Autodesk Inventor part; units mm, degrees
ref_plane "YZ Plane" through (0, 0, 0) normal (1, 0, 0) x (0, 1, 0)
ref_plane "XZ Plane" through (0, 0, 0) normal (0, 1, 0) x (-1, 0, 0)
ref_plane "XY Plane" through (0, 0, 0) normal (0, 0, 1) x (1, 0, 0)
sketch "Sketch1" plane through (0, 0, 0) normal (0, 0, 1) x (1, 0, 0)
  line L0 (0, 0) -> (189.177, 0)
  line L1 (189.177, 0) -> (189.177, 325.825)
  line L2 (189.177, 325.825) -> (0, 325.825)
  line L3 (0, 325.825) -> (0, 0)
  dimension "d0" = 189.177
  dimension "d1" = 325.825
extrude "Extrusion1" add sketch "Sketch1" along normal blind 2.6
sketch "Sketch2" plane through (0, 0, 2.6) normal (0, 0, 1) x (1, 0, 0)
  line L0 (0, 325.825) -> (0, 0)
  line L1 (0, 170) -> (0, 0)
  line L2 (0, 170) -> (0, 159.84) construction
  line L3 (0, 159.84) -> (6.35, 159.84) construction
  line L4 (6.35, 170) -> (163.83, 170) construction
  line L5 (163.83, 170) -> (163.83, 136.98) construction
  line L6 (6.35, 159.84) -> (6.35, 4.9) construction
  line L7 (6.35, 4.9) -> (163.83, 4.9) construction
  line L8 (6.35, 159.84) -> (15.9385, 159.84) construction
  line L9 (15.9385, 159.84) -> (15.9385, 4.9) construction
  line L10 (163.83, 136.98) -> (173.4185, 136.98) construction
  line L11 (173.4185, 136.98) -> (173.4185, 4.9) construction
  line L12 (0, 325.825) -> (0, 315.665) construction
  line L13 (15.9385, 159.84) -> (15.9385, 315.665) construction
  line L14 (173.4185, 136.98) -> (173.4185, 292.805) construction
  line L15 (15.9385, 4.9) -> (15.9385, 160.725) construction
  line L16 (173.4185, 4.9) -> (173.4185, 160.725) construction
  circle A0 centre (173.4185, 160.725) radius 1.98
  circle A1 centre (15.9385, 160.725) radius 1.98
  circle A2 centre (15.9385, 315.665) radius 1.98
  circle A3 centre (173.4185, 292.805) radius 1.98
  dimension "d4" = 10.16
  dimension "d6" = 157.48
  dimension "d7" = 33.02
  dimension "d8" = 154.94
  dimension "d13" = 9.5885
  dimension "d14" = 9.5885
  dimension "d19" = 10.16
  dimension "d20" = 155.825
  dimension "d21" = 155.825
  dimension "d22" = 155.825
  dimension "d23" = 3.96
  dimension "d24" = 3.96
  dimension "d25" = 3.96
  dimension "d26" = 3.96
extrude "Extrusion2" cut sketch "Sketch2" against normal blind 5
sketch "Sketch4" plane through (0, 0, 2.6) normal (0, 0, 1) x (1, 0, 0)
  line L0 (0, 0) -> (189.177, 0)
  line L1 (189.177, 0) -> (164.5885, 0) construction
  line L2 (164.5885, 0) -> (24.5885, 0)
  line L3 (24.5885, 0) -> (24.5885, 40)
  line L4 (24.5885, 40) -> (164.5885, 40)
  line L5 (164.5885, 40) -> (164.5885, 0)
  dimension "d29" = 24.5885
  dimension "d30" = 140
  dimension "d31" = 40
extrude "Extrusion3" cut sketch "Sketch4" against normal blind 10
properties part number "trunk"
Geometry check sheet. Reference: the model listing, model coordinates, mm. Coordinates: 2 decimals unless noted, no trailing zeros. Write each loop counter-clockwise with the first axis right and the second up, starting at its lowest first coordinate (ties: lowest second). Pieces come first, ordered by that corner, then holes. Notation, with made-up numbers: M 47.25,76 L 57.25,76 A36 ccw 57.25,115 Z; hole C 51.5,82 d10. An arc over 180 degrees is marked long. One line per item, written item: value. Start each with the question number.
(1) Sectioned sample at B-B, the plane x = 60. Enter the section's corners in (y, z) (3 decimals).
(2) Sectioned sample at A-A, the plane z = 1.7. Enter the section's corners in (x, y) (1 decimal), and give its area (3 significant figures).
(3) Depth check by flat-ended pin: pin 1 (1.3 mm diameter, centred on x = 105, z = 1.5, fed in from -Y). Enter the tip coordinate at first touch or a pass-through.
(4) Scan lines: line 1 along X through (y, z) = (22.5, 2.2); line 2 along Y through (x, z) = (175, 0.6) (3 decimals); line 3 along Y through (x, z) = (33, 0.45) (3 decimals). Record each from-to range of solid material in increasing order. Write a range as [from, to].
Filled sheet:
1. outline: M 40,0 L 325.825,0 L 325.825,2.6 L 40,2.6 Z
2. outline: M 0,0 L 24.6,0 L 24.6,40 L 164.6,40 L 164.6,0 L 189.2,0 L 189.2,325.8 L 0,325.8 Z; hole C 15.9,160.7 d4; hole C 15.9,315.7 d4; hole C 173.4,160.7 d4; hole C 173.4,292.8 d4
2. area: 56,000 mm²
3. pin 1: y = 40
4. line 1: [0, 24.59], [164.59, 189.18]
4. line 2: [0, 159.534], [161.916, 291.614], [293.996, 325.825]
4. line 3: [40, 325.825]
